The listing builds one solid part. Answer for the finished solid, in the listing's coordinates (mm). A direction names the side the tool comes from. Give positions to 0.01 mm unless a question says otherwise; leave off trailing zeros. Loops run counter-clockwise (first coordinate to the right, second up) from the corner with the lowest first, then second, coordinate; pieces in that order, holes last. Notation, with made-up numbers: (75.5, 35.5) - (88.5, 35.5) arc R19 ccw to (88.5, 51.5) - close; hole circle Ø2 at (-26, 30.25). An arc over 180 degrees is marked (long way). Answer as CSV lines item,"result". Start each with the question number.
1) A cutting plane is placed at A-A (x = 0). Determine the outline of the cut face in (y, z) (3 decimals).
2) Flat-ended cylindrical pins translate along their axes: pin 1 (3.5 mm diameter, centred on y = 2.5, z = 1.5, fed in from +X); pin 2 (4 mm diameter, centred on y = 55.5, z = 4.5, fed in from +X); pin 3 (2.5 mm diameter, centred on x = 0, y = 31.905, fed in from -Z); pin 4 (4.5 mm diameter, centred on x = 1, y = 31, fed in from -Z). Find the tip coordinate at first contact, or state that the pin passes through.
3) A cutting plane is placed at B-B (z = 0). Determine the outline of the cut face in (x, y) (3 decimals).
4) For a pull along Y with two mould halves and no side action, classify faces 5 (the face through (3.75, 33, 9)), 6 (the face through (-2, 7.75, 2)), 7 (the face through (1.695, 61.014, 7.116)) as pulls with the +Y half, pulls with the -Y half, needs draft (parallel to the pull), parting line crosses it, or undercut.
5) Find the intervals of material crossed by line 1 along Y through (x, z) = (0, 11.1) (3 decimals); line 2 along Y through (x, z) = (2, 6.75); line 3 along Z through (x, y) = (1, 19), in increasing order.
6) A cutting plane is placed at C-C (y = 17.5). Determine the outline of the cut face in (x, z).
7) For faces 1 (the face through (-3.25, 4, 0)), 2 (the face through (3.25, 4, 0)), 3 (the face through (0, 38, 6.13)), 4 (the face through (0, 60.026, 7)), determine the directions among +Z, -Z, +X, -X, +Y, -Y from which every point of the face is accessible in a straight line to the end or side of a thin tool.
```python
from build123d import *

# Parameters (mm, degrees)
SKETCH1_W           = 6.5
SKETCH1_H           = 6.5
SKETCH1_R           = 2.625
BOSS_EXTRUDE1_DEPTH = 7.75
SKETCH2_W           = 6.5
SKETCH2_H           = 7.75
BOSS_EXTRUDE2_DEPTH = 8.88
SKETCH3_W           = 6.5
SKETCH3_H           = 6
BOSS_EXTRUDE3_DEPTH = 58.01
FILLET1_R           = 2.5
BOSS_EXTRUDE4_START = 0.5
BOSS_EXTRUDE4_DEPTH = 0.5
FILLET2_R           = 0.5
FILLET3_R           = 0.5
SKETCH6_R           = 1
CUT_EXTRUDE3_DEPTH  = 67.53137982
CUT_EXTRUDE4_DEPTH  = 2


with BuildPart() as part:
    # Sketch1 → Boss-Extrude1 (new body)
    with BuildSketch(Plane(origin=(0, 0, 0), x_dir=(1, 0, 0), z_dir=(0, 1, 0))):
        Rectangle(SKETCH1_W, SKETCH1_H)
        with Locations(Location((0, 0, 0), (0, 0, 270))):
            Circle(SKETCH1_R, mode=Mode.SUBTRACT)
    extrude(amount=BOSS_EXTRUDE1_DEPTH)

    # Sketch2 → Boss-Extrude2 (add)
    with BuildSketch(Plane.XY.offset(3.25)):
        with Locations((0, 3.875)):
            Rectangle(SKETCH2_W, SKETCH2_H)
    extrude(amount=BOSS_EXTRUDE2_DEPTH)

    # Sketch3 → Boss-Extrude3 (add)
    with BuildSketch(Plane(origin=(0, 7.75, 0), x_dir=(1, 0, 0), z_dir=(0, 1, 0))):
        with Locations((0, -9.13)):
            Rectangle(SKETCH3_W, SKETCH3_H)
    extrude(amount=BOSS_EXTRUDE3_DEPTH)

    # Fillet1
    fillet1_edges = [part.edges().sort_by_distance(p)[0] for p in [
        (0, 7.75, 6.13),
    ]]
    fillet(fillet1_edges, radius=FILLET1_R)

    # Sketch4 → Boss-Extrude4 (add)
    with BuildSketch(Plane(origin=(3.25, 0, 0), x_dir=(0, 0, -1), z_dir=(1, 0, 0)).offset(BOSS_EXTRUDE4_START)):
        with BuildLine():
            Line((-3.63, 7.75), (-3.63, 0))
            Line((-3.63, 0), (-12.13, 0))
            Line((-12.13, 0), (-12.13, 65.76))
            Line((-12.13, 65.76), (-6.13, 65.76))
            Line((-6.13, 65.76), (-6.13, 10.25))
            ThreePointArc((-6.13, 10.25), (-5.397766953, 8.482233047), (-3.63, 7.75))
        make_face()
    boss_extrude4 = extrude(amount=-BOSS_EXTRUDE4_DEPTH)

    # Fillet2
    fillet2_edges = [part.edges().sort_by_distance(p)[0] for p in [
        (3.75, 3.875, 3.63),
    ]]
    fillet(fillet2_edges, radius=FILLET2_R - 0.0001)  # a hair under: the kernel refuses the full size

    # Mirror1: Boss-Extrude4 across plane
    add(boss_extrude4.mirror(Plane(origin=(0, 0, 0), x_dir=(0, 0, 1), z_dir=(1, 0, 0))))

    # Fillet3
    fillet3_edges = [part.edges().sort_by_distance(p)[0] for p in [
        (-3.75, 3.875, 3.63),
    ]]
    fillet(fillet3_edges, radius=FILLET3_R - 0.0001)  # a hair under: the kernel refuses the full size

    # Sketch6 → Cut-Extrude3 (cut, through all)
    with BuildSketch(Plane(origin=(0, 0, 6.13), x_dir=(-1, 0, 0), z_dir=(0, 0, -1))):
        with Locations((0, 61.975)):
            Circle(SKETCH6_R)
    cut_extrude3 = extrude(amount=-CUT_EXTRUDE3_DEPTH, mode=Mode.SUBTRACT)

    # Sketch6<3> → Cut-Extrude4 (cut)
    with BuildSketch(Plane(origin=(0, 0, 6.13), x_dir=(-1, 0, 0), z_dir=(0, 0, -1))):
        Polygon((2.25, 61.975), (1.125, 63.923557159), (-1.125, 63.923557159), (-2.25, 61.975), (-1.125, 60.026442841), (1.125, 60.026442841), align=None)
    cut_extrude4 = extrude(amount=-CUT_EXTRUDE4_DEPTH, mode=Mode.SUBTRACT)

    # Mirror2: Cut-Extrude3, Cut-Extrude4 across plane
    add(cut_extrude3.mirror(Plane.ZX.offset(46.94)), mode=Mode.SUBTRACT)
    add(cut_extrude4.mirror(Plane.ZX.offset(46.94)), mode=Mode.SUBTRACT)


solid = part.part
```
Ans:
1,outline,"(0, -3.25) - (7.75, -3.25) - (7.75, -2.625) - (0, -2.625) - close; (0, 2.625) - (7.75, 2.625) - (7.75, 3.63) arc R2.5 cw to (10.25, 6.13) - (29.956, 6.13) - (29.956, 8.13) - (30.905, 8.13) - (30.905, 12.13) - (0, 12.13) - close; (32.905, 8.13) - (33.854, 8.13) - (33.854, 6.13) - (60.026, 6.13) - (60.026, 8.13) - (60.975, 8.13) - (60.975, 12.13) - (32.905, 12.13) - close; (62.975, 8.13) - (63.924, 8.13) - (63.924, 6.13) - (65.76, 6.13) - (65.76, 12.13) - (62.975, 12.13) - close"
2,pin 1,"x = 3.25"
2,pin 2,"x = 3.75"
2,pin 3,"z = 8.13"
2,pin 4,"z = 6.13"
3,outline,"(-3.25, 0) - (-2.625, 0) - (-2.625, 7.75) - (-3.25, 7.75) - close; (2.625, 0) - (3.25, 0) - (3.25, 7.75) - (2.625, 7.75) - close"
4,face 5,"needs draft"
4,face 6,"pulls with the +Y half"
4,face 7,"undercut"
5,line 1,"0 to 30.905, 32.905 to 60.975, 62.975 to 65.76"
5,line 2,"0 to 31.47, 32.34 to 61.54, 62.41 to 65.76"
5,line 3,"6.13 to 12.13"
6,outline,"(-3.75, 6.13) - (3.75, 6.13) - (3.75, 12.13) - (-3.75, 12.13) - close"
7,face 1,"-Z, -X, +Y, -Y"
7,face 2,"-Z, +X, +Y, -Y"
7,face 3,"-Z, +X, -X, +Y"
7,face 4,"-Z"
